from build123d import *

# Parameters (mm, degrees)
BOSS_EXTRUDE1_DEPTH              = 5
BOSS_EXTRUDE2_DEPTH              = 13
CUT_EXTRUDE1_START               = -13
SKETCH3_R                        = 2.3
CUT_EXTRUDE1_DEPTH               = 7.5
CUT_EXTRUDE2_DEPTH               = 57.683541142
CUT_EXTRUDE2_DEPTH_BACK          = 57.683541142
CBORE_FOR_M2_5_SHCS1_D           = 2.9
CBORE_FOR_M2_5_SHCS1_CBORE_D     = 5
CBORE_FOR_M2_5_SHCS1_CBORE_DEPTH = 13.5


with BuildPart() as part:
    # Sketch1 → Boss-Extrude1 (new body)
    with BuildSketch(Plane(origin=(0, 0, 0), x_dir=(0, 0, -1), z_dir=(1, 0, 0))):
        with BuildLine():
            Line((-34.593659354, 3.256520294), (-46.7897518, -6.296129983))
            ThreePointArc((-46.7897518, -6.296129983), (-33.290290023, -15.004245976), (-18.234604608, -20.60719958))
            Line((-18.234604608, -20.60719958), (-2.973495544, 21.32235297))
            Line((-2.973495544, 21.32235297), (-17.068884855, 26.45265512))
            Line((-17.068884855, 26.45265512), (-27.166620772, -1.290646299))
            ThreePointArc((-27.166620772, -1.290646299), (-30.963724442, 0.846415848), (-34.593659354, 3.256520294))
        make_face()
    extrude(amount=BOSS_EXTRUDE1_DEPTH)

    # Sketch2 → Boss-Extrude2 (add)
    with BuildSketch(Plane(origin=(5, 0, 0), x_dir=(0, 0, -1), z_dir=(1, 0, 0))):
        with BuildLine():
            Line((-34.593659354, 3.256520294), (-46.7897518, -6.296129983))
            ThreePointArc((-46.7897518, -6.296129983), (-42.613802597, -9.444548196), (-38.226724688, -12.291412509))
            Line((-38.226724688, -12.291412509), (-25.335917908, -2.194623762))
            ThreePointArc((-25.335917908, -2.194623762), (-26.255160174, -1.750514609), (-27.166620772, -1.290646299))
            ThreePointArc((-27.166620772, -1.290646299), (-30.963724442, 0.846415848), (-34.593659354, 3.256520294))
        make_face()
        with BuildLine():
            Line((-25.335917908, -2.194623762), (-38.226724688, -12.291412509))
            ThreePointArc((-38.226724688, -12.291412509), (-28.535215176, -17.181480963), (-18.234604608, -20.60719958))
            Line((-18.234604608, -20.60719958), (-12.16072752, -3.919359432))
            Line((-12.16072752, -3.919359432), (-2.973495544, 21.32235297))
            Line((-2.973495544, 21.32235297), (-17.068884855, 26.45265512))
            Line((-17.068884855, 26.45265512), (-26.256116832, 1.210942718))
            Line((-26.256116832, 1.210942718), (-27.166620772, -1.290646299))
            ThreePointArc((-27.166620772, -1.290646299), (-26.255160174, -1.750514609), (-25.335917908, -2.194623762))
        make_face()
    extrude(amount=BOSS_EXTRUDE2_DEPTH)

    # Sketch3 → Cut-Extrude1 (cut)
    with BuildSketch(Plane(origin=(18, 0, 0), x_dir=(0, 0, -1), z_dir=(1, 0, 0)).offset(CUT_EXTRUDE1_START)):
        with Locations((-40.691705577, -1.519804845)):
            Circle(SKETCH3_R)
    extrude(amount=CUT_EXTRUDE1_DEPTH, mode=Mode.SUBTRACT)

    # Sketch8 → Cut-Extrude2 (cut, two sides: drawn at the far end of the back side and taken through both)
    with BuildSketch(Plane.ZY.offset(-CUT_EXTRUDE2_DEPTH_BACK)):
        with BuildLine():
            Line((27.166620772, -1.290646299), (17.068884855, 26.45265512))
            Line((17.068884855, 26.45265512), (2.973495544, 21.32235297))
            Line((2.973495544, 21.32235297), (17.068884855, -17.404410883))
            Line((17.068884855, -17.404410883), (17.068884855, -5.36984615))
            ThreePointArc((17.068884855, -5.36984615), (22.211595111, -3.562545394), (27.166620772, -1.290646299))
        make_face()
    extrude(amount=CUT_EXTRUDE2_DEPTH + CUT_EXTRUDE2_DEPTH_BACK, mode=Mode.SUBTRACT)

    # CBORE for M2.5 SHCS1 (through all)
    with Locations(Plane(origin=(18, 0, 0), x_dir=(0, 0, -1), z_dir=(1, 0, 0))):
        with Locations((-37.335347169, -3.97184687), (-24.568884855, -6.047927384), (-21.576904852, -15.17107203)):
            CounterBoreHole(CBORE_FOR_M2_5_SHCS1_D / 2, CBORE_FOR_M2_5_SHCS1_CBORE_D / 2, CBORE_FOR_M2_5_SHCS1_CBORE_DEPTH)


solid = part.part
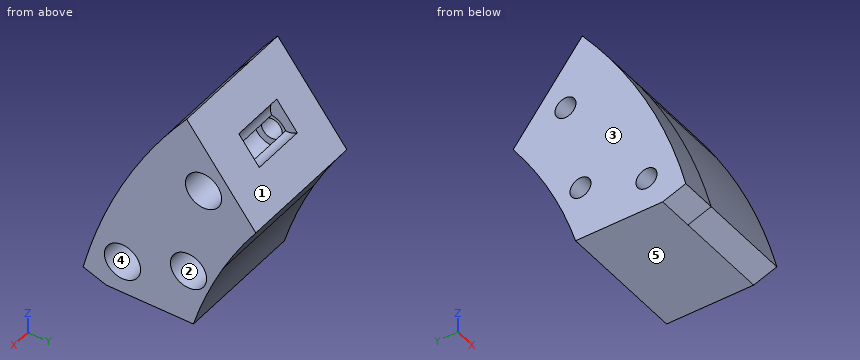
The model under review builds one solid part; all positions refer to its coordinate system, in mm. Face numbers are marked on the shaded views. A direction names the side the tool comes from. Round coordinates to 2 decimals unless told otherwise and drop trailing zeros. Write each loop counter-clockwise with the first axis right and the second up, starting at its lowest first coordinate (ties: lowest second). Pieces come first, ordered by that corner, then holes. Notation, with made-up numbers: (-35.75, 48.5) - (9.25, 48.5) arc R32 cw to (9.25, 78.5) - close; hole circle Ø7 at (21.25, -10.75). An arc over 180 degrees is marked (long way). One line per item, written item: value. Start each with the question number.
1. Consider section D-D on x = 10.75. Write out the cut boundary in (y, z).
2. Machinability: for the marked faces 4 and 5, which of the approach directions +Z, -Z, +X, -X, +Y, -Y give a long, thin tool a straight path to every point of the face, cutting with its end or side? Answer none if there is none.
3. Consider section C-C on x = 3. Write out the cut boundary in (y, z).
4. The part is to be moulded in two halves that separate along Y. For the marked faces 1, 2 and 3, say which applies: released by +Y, released by -Y, zero draft, split by the parting line, or undercut.
5. Consider section A-A on y = -14.25. Write out the cut boundary in (x, z).
6. To check wall thickness, follow L1, parallel to Y at x = 9.5, z = 22.5; L2, parallel to Z at x = 6.5, y = -15; L3, parallel to X at y = -4.5, z = 39.25. State the ranges of each line that lie inside material, in increasing order. Write a range as from..to.
7. Consider section B-B on z = 25. Write out the cut boundary in (x, y).
8. Clearance check with flat-ended pins moving along their axes: P1, Ø4, axis at y = -3.97, z = 37.34, coming from the +X side; P2, Ø3, axis at x = 6, z = 31.5, coming from the -Y side; P3, Ø2, axis at x = 14.5, z = 24.5, coming from the -Y side. State where each tip first meets the part, or that it passes through.
Checks:
1. outline: (-20.61, 18.23) - (-17.4, 17.07) - (-5.37, 17.07) arc R59.3 cw to (3.26, 34.59) - (-0.1, 38.88) arc R2.3 cw to (-1.71, 38.4) arc R2.5 cw (long way) to (-3.65, 39.81) arc R2.3 cw to (-2.94, 42.5) - (-6.3, 46.79) arc R74.3 ccw to start; hole circle Ø5 at (-15.17, 21.58); hole circle Ø5 at (-6.05, 24.57)
2. face 4: +X
2. face 5: -Z, +X, -X, +Y, -Y
3. outline: (-20.61, 18.23) - (-17.4, 17.07) - (-5.37, 17.07) arc R59.3 cw to (3.26, 34.59) - (-6.3, 46.79) arc R74.3 ccw to start; hole circle Ø2.9 at (-15.17, 21.58); hole circle Ø2.9 at (-6.05, 24.57); hole circle Ø2.9 at (-3.97, 37.34)
4. face 1: released by +Y
4. face 2: undercut
4. face 3: zero draft
5. outline: (0, 17.07) - (18, 17.07) - (18, 19.25) - (4.5, 19.25) - (4.5, 20.46) - (0, 20.46) - close; (0, 22.7) - (4.5, 22.7) - (4.5, 23.9) - (18, 23.9) - (18, 34.75) - (0, 34.75) - close
6. L1: y = -19.39..-17.49, -12.85..-7.45, -4.64..-3.45
6. L2: z = 17.07..19.08, 24.07..33.3
6. L3: x = 0..4.5
7. outline: (0, -18.55) - (18, -18.55) - (18, -8.51) - (4.5, -8.51) - (4.5, -7.43) - (0, -7.43) - close; (0, -4.66) - (4.5, -4.66) - (4.5, -3.59) - (18, -3.59) - (18, -2.35) - (0, -2.35) - close
8. P1: stops at x = 4.5
8. P2: stops at y = -16.55
8. P3: stops at y = -19.07
